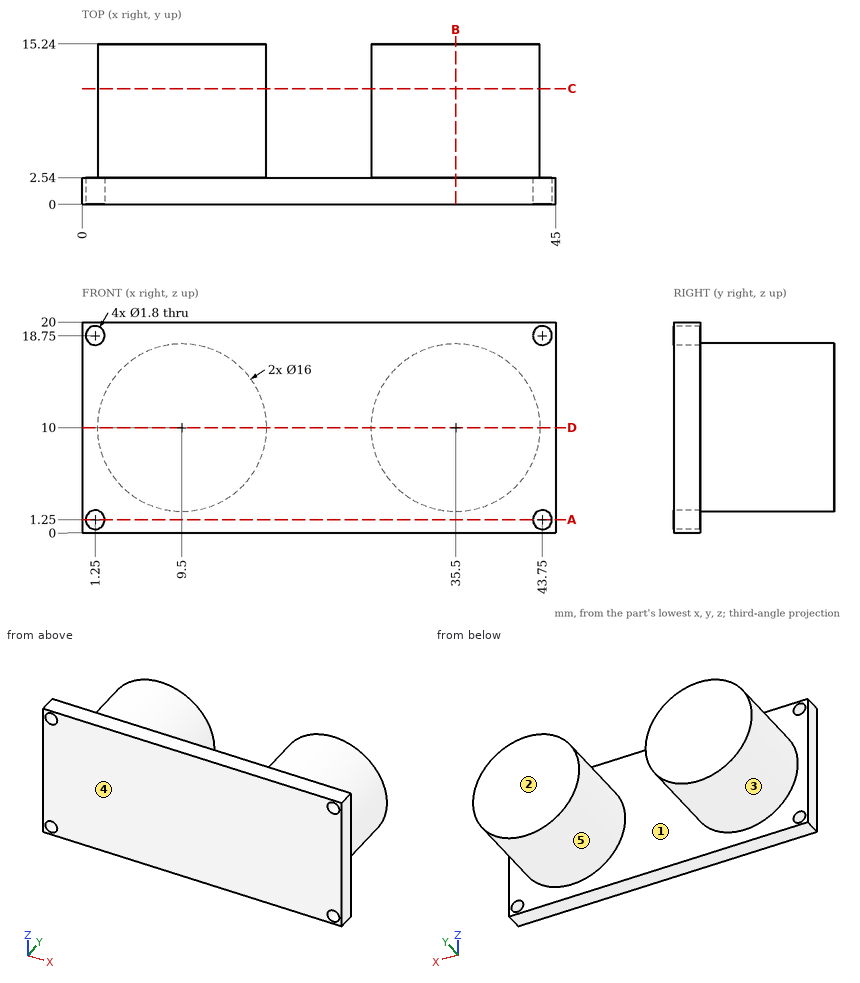
Design review of the part shown in the three views and the two pictorial views. Dimensions are in mm from the part's minimum x, y and z. A direction names the side the tool comes from. Give positions to 0.01 mm unless a question says otherwise; leave off trailing zeros. Write each loop counter-clockwise with the first axis right and the second up, starting at its lowest first coordinate (ties: lowest second). Pieces come first, ordered by that corner, then holes.
(1) Clearance check with flat-ended pins moving along their axes: pin 1 Ø8 at (x, y) = (17.5, 7) entering from +Z; pin 2 Ø3 at (x, z) = (43.75, 18.75) entering from +Y; pin 3 Ø4 at (x, y) = (14, 5) entering from +Z. State where each tip first meets the part, or that it passes through.
Checked values:
pin 1: stops at z = 16.93
pin 2: stops at y = 2.54
pin 3: stops at z = 17.6
(2) Tool access review of the marked faces 4 and 5: name each direction out of +Z, -Z, +X, -X, +Y, -Y from which nothing blocks a thin tool from reaching the whole face with its end or side.
Checked values:
face 4: +Z, -Z, +X, -X, -Y
face 5: +Y
(3) Mouldability with a two-part tool opening along X and no side actions: class the marked faces 1, 2 and 3 as +X half, -X half, draft (parallel to the pull), parting line (faces both ways), or undercut.
Checked values:
face 1: undercut
face 2: draft
face 3: undercut
(4) Wall thickness on line 1 along X through (y, z) = (0.7, 1.25); line 2 along Z through (x, y) = (43.75, 1.9); line 3 along X through (y, z) = (4, 10): over which ranges is each line inside the solid? List them lowest first.
Checked values:
line 1: x = 0 to 0.35, 2.15 to 42.85, 44.65 to 45
line 2: z = 0 to 0.35, 2.15 to 17.85, 19.65 to 20
line 3: x = 1.5 to 17.5, 27.5 to 43.5
(5) Add section D-D (z = 10). Give the boundary of the cut face in (x, y).
Checked values:
outline: (0, 0) - (45, 0) - (45, 2.54) - (43.5, 2.54) - (43.5, 15.24) - (27.5, 15.24) - (27.5, 2.54) - (17.5, 2.54) - (17.5, 15.24) - (1.5, 15.24) - (1.5, 2.54) - (0, 2.54) - close
(6) Add section C-C (y = 11). Give the boundary of the cut face in (x, z).
Checked values:
outline: circle Ø16 at (9.5, 10); circle Ø16 at (35.5, 10)
(7) Add section B-B (x = 35.5). Give the boundary of the cut face in (y, z), and give its area (3 significant figures).
Checked values:
outline: (0, 0) - (2.54, 0) - (2.54, 2) - (15.24, 2) - (15.24, 18) - (2.54, 18) - (2.54, 20) - (0, 20) - close
area: 254 mm2
(8) Add section A-A (z = 1.25). Give the boundary of the cut face in (x, y).
Checked values:
outline: (0, 0) - (0.35, 0) - (0.35, 2.54) - (0, 2.54) - close; (2.15, 0) - (42.85, 0) - (42.85, 2.54) - (2.15, 2.54) - close; (44.65, 0) - (45, 0) - (45, 2.54) - (44.65, 2.54) - close
